Answer from the drawing. Dimensions are ordinates in mm from the lowest x, y and z of the part. A direction names the side the tool comes from. Give positions to 0.01 mm unless a question says otherwise; leave off trailing zeros. Write each loop counter-clockwise with the first axis right and the second up, starting at its lowest first coordinate (ties: lowest second). Pieces come first, ordered by that corner, then holes.
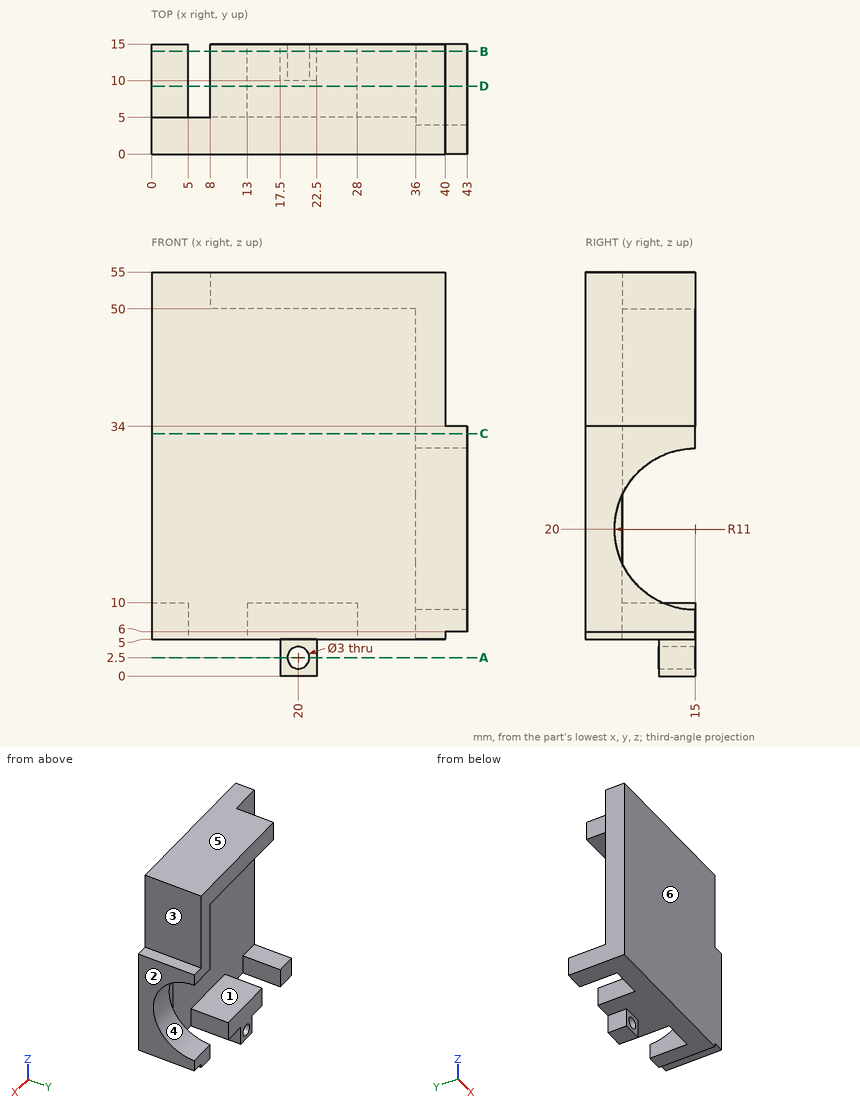
Item 1: A cutting plane is placed at C-C, the plane z = 33. Give the vertices of the cut face in (x, y), plus the area to 3 significant figures.
Conclusion:
outline: (0, 0) - (43, 0) - (43, 15) - (36, 15) - (36, 5) - (0, 5) - close
area: 285 mm2
Item 2: A cutting plane is placed at B-B, the plane y = 14. Give the vertices of the cut face in (x, z).
Conclusion:
outline: (0, 5) - (5, 5) - (5, 10) - (0, 10) - close; (8, 50) - (36, 50) - (36, 30.95) - (43, 30.95) - (43, 34) - (40, 34) - (40, 55) - (8, 55) - close; (13, 5) - (17.5, 5) - (17.5, 0) - (22.5, 0) - (22.5, 5) - (28, 5) - (28, 10) - (13, 10) - close; (36, 5) - (40, 5) - (40, 6) - (43, 6) - (43, 9.05) - (36, 9.05) - close; hole circle Ø3 at (20, 2.5)
Item 3: Which of the six approach directions +Z, -Z, +X, -X, +Y, -Y give full straight-line access (tool end or side, diameter ignored) to the marked faces 1, 2 and 3?
Conclusion:
face 1: -X, +Y
face 2: +Z, -Z, +X, +Y, -Y
face 3: +Z, +X, +Y, -Y
Item 4: A cutting plane is placed at A-A, the plane z = 2.5. Give the vertices of the cut face in (x, y).
Conclusion:
outline: (17.5, 10) - (18.5, 10) - (18.5, 15) - (17.5, 15) - close; (21.5, 10) - (22.5, 10) - (22.5, 15) - (21.5, 15) - close
Item 5: Determine the mould class of the marked faces 4, 5 and 6 for opening direction Z: pulls with the +Z half, pulls with the -Z half, needs draft (parallel to the pull), parting line crosses it, or undercut.
Conclusion:
face 4: undercut
face 5: pulls with the +Z half
face 6: needs draft
Item 6: A cutting plane is placed at D-D, the plane y = 9.25. Give the vertices of the cut face in (x, z), plus the area to 3 significant figures.
Conclusion:
outline: (0, 5) - (5, 5) - (5, 10) - (0, 10) - close; (8, 50) - (36, 50) - (36, 29.38) - (43, 29.38) - (43, 34) - (40, 34) - (40, 55) - (8, 55) - close; (13, 5) - (28, 5) - (28, 10) - (13, 10) - close; (36, 5) - (40, 5) - (40, 6) - (43, 6) - (43, 10.62) - (36, 10.62) - close
area: 393 mm2
Item 7: Consider probe 1 along X at (y, z) = (5.75, 5.5); probe 2 along X at (y, z) = (11.7, 2.5); probe 3 along Z at (x, y) = (15, 13). Determine where each line is inside the solid, lowest interval first.
Conclusion:
probe 1: x = 0 to 5, 13 to 28, 36 to 40
probe 2: x = 17.5 to 18.5, 21.5 to 22.5
probe 3: z = 5 to 10, 50 to 55
Item 8: Each of these flat-tipped pins is pushed along its axis until it touches: P1, Ø6, axis at x = 25.5, z = 40, coming from the +Y side; P2, Ø2.5, axis at x = 3.5, y = 9.5, coming from the +Z side; P3, Ø4, axis at y = 9, z = 52, coming from the -X side. Where does it stop, or does it pass through?
Conclusion:
P1: stops at y = 5
P2: stops at z = 10
P3: stops at x = 8
